Read the model definition and answer for the solid it produces. Units are mm, in the model's axes. A direction names the side the tool comes from. Coordinates: 2 decimals unless noted, no trailing zeros. Write each loop counter-clockwise with the first axis right and the second up, starting at its lowest first coordinate (ties: lowest second). Pieces come first, ordered by that corner, then holes.
Item 1: Straight lines are drawn through the part: probe 1 along Y at (x, z) = (2, 16.5); probe 2 along Y at (x, z) = (-1, 15); probe 3 along Z at (x, y) = (11, 477.5). For each, find the intervals that lie inside material, in ascending order.
Item 2: Section A-A (y = 910) is taken. Give the vertices of the cut face in (x, z), then the cut area to 3 significant figures.
Item 3: Section B-B (y = 131) is taken. Give the vertices of the cut face in (x, z), then the cut area to 3 significant figures.
Item 4: Determine the mould class of faces 1 (the face through (-19.524, 122.157, -4.336)), 2 (the face through (-14.2, 374.12, 7.7)), 3 (the face through (-8, -21.88, 11)) for opening direction Y: released by +Y, released by -Y, zero draft, split by the parting line, or undercut.
Item 5: Each of these flat-tipped pins is pushed along its axis until it touches: P1, Ø1, axis at x = -2.5, y = 438, coming from the +Z side; P2, Ø3, axis at x = -8, y = 683.5, coming from the -Z side; P3, Ø4, axis at x = 2, y = -47.5, coming from the +Z side. Where does it stop, or does it pass through?
Item 6: A tool of negligible diameter and unlimited length cuts with its end or side. For faces 4 (the face through (8.45, -42.16, -9.21)), 5 (the face through (-18, 228.12, 0)), 6 (the face through (-14, 706, 0)), 7 (the face through (-6.32, -8.69, 15.24)), from which of +Z, -Z, +X, -X, +Y, -Y can it reach the whole face along a straight path? Write none if from no direction.
from build123d import *

# Parameters (mm, degrees)
F3_DEPTH = 33
F0_W     = 575
F0_H     = 17.5
F7_DEPTH = 575


with BuildPart() as f1:
    # F0 (on Right) → F1 (revolve)
    with BuildSketch(Plane.YZ):
        Polygon((-9.479858, 17.5), (-21.879858, 17.5), (-21.879858, 12.5), (-61.879858, 12.5), (-61.879858, 0), (-21.879858, 0), (19.120142, 0), (19.120142, 17.5), (-7.879858, 17.5), (-7.879858, 16.5), (-9.479858, 16.5), align=None)
    revolve(axis=Axis((0, 215.2909, 0), (0, 1, 0)))

    # F2 (on face) → F3 (cut)
    with BuildSketch(Plane.XZ.offset(61.879858)):
        with BuildLine():
            ThreePointArc((6.78233, 10.5), (0, 12.5), (-6.78233, 10.5))
            Line((-6.78233, 10.5), (6.78233, 10.5))
        make_face()
        with BuildLine():
            Line((6.78233, -10.5), (-6.78233, -10.5))
            ThreePointArc((-6.78233, -10.5), (0, -12.5), (6.78233, -10.5))
        make_face()
    extrude(amount=-F3_DEPTH, mode=Mode.SUBTRACT)

    # F0 (on Right) → F4 (revolve)
    with BuildSketch(Plane.YZ):
        Polygon((19.120142, 20), (19.120142, 17.5), (19.120142, 0), (414.120142, 0), (414.120142, 17.5), (401.720142, 17.5), (401.720142, 13.727913), (400.120142, 13.727913), (400.120142, 17.5), (374.120142, 17.5), (374.120142, 16), (261.120142, 16), (261.120142, 17.5), (228.120142, 17.5), (228.120142, 20), align=None)
    revolve(axis=Axis((0, 216.620142, 0), (0, 1, 0)))

    # F0 (on Right) → F5 (revolve)
    with BuildSketch(Plane.YZ):
        with Locations((701.620142, 8.75)):
            Rectangle(F0_W, F0_H)
    revolve(axis=Axis((0, 701.620142, 0), (0, 1, 0)))

    # F6 (on face) → F7 (cut)
    with BuildSketch(Plane(origin=(0, 989.120142, 0), x_dir=(-1, 0, 0), z_dir=(0, 1, 0))):
        with BuildLine():
            ThreePointArc((17.5, 0), (16.601958, 5.533986), (14, 10.5))
            Line((14, 10.5), (14, -10.5))
            ThreePointArc((14, -10.5), (16.601958, -5.533986), (17.5, 0))
        make_face()
        with BuildLine():
            Line((-14, -10.5), (-14, 10.5))
            ThreePointArc((-14, 10.5), (-17.5, 0), (-14, -10.5))
        make_face()
    extrude(amount=-F7_DEPTH, mode=Mode.SUBTRACT)


solid = f1.part
Established:
1. probe 1: y = -21.88 to -9.48, -7.88 to 261.12, 374.12 to 400.12, 401.72 to 989.12
1. probe 2: y = -21.88 to 400.12, 401.72 to 989.12
1. probe 3: z = -13.61 to 13.61
2. outline: (-14, -10.5) arc R17.5 ccw to (14, -10.5) - (14, 10.5) arc R17.5 ccw to (-14, 10.5) - close
2. area: 862 mm2
3. outline: circle Ø40 at (0, 0)
3. area: 1,260 mm2
4. face 1: zero draft
4. face 2: undercut
4. face 3: released by -Y
5. P1: stops at z = 17.39
5. P2: stops at z = -16.25
5. P3: stops at z = 10.5
6. face 4: -Y
6. face 5: +Y
6. face 6: +Z, -Z, -X, +Y
6. face 7: none
